Geometry: final body of the model. Coordinates: model frame, mm. A direction names the side the tool comes from. Coordinates: 2 decimals unless noted, no trailing zeros. Write each loop counter-clockwise with the first axis right and the second up, starting at its lowest first coordinate (ties: lowest second). Pieces come first, ordered by that corner, then holes. Notation, with made-up numbers: (-23.75, 77) - (12.25, 77) arc R27 ccw to (12.25, 113) - close; hole circle Ø10 at (51.25, 15). An arc over 180 degrees is marked (long way). Answer as a JSON object with one key per item and string values. Group by question number.
Item 1: Section B-B on y = -5. Return loops of the section in (x, z).
Item 2: Mould query, pull axis X, two halves, no side actions, for faces 1 (the flat face through (28, 0, -11)), 2 (the flat face through (-20, 0, -4)), 3 (the cylindrical face through (-22.7, -5.8, -10.6)). Classes: pulls with the +X half, pulls with the -X half, needs draft (parallel to the pull), parting line crosses it, or undercut.
Item 3: First-contact query: pin 1 Ø4 at (x, y) = (-25.5, 4) entering from -Z; pin 2 Ø10 at (y, z) = (4.5, -25.5) entering from +X; pin 3 Ø10 at (x, y) = (9, 1.5) entering from +Z. Flat tips, straight axial feed; report the tip coordinate or a pass-through.
Item 4: Set-up query: faces 4 (the cylindrical face through (0, 0, 3)), 5 (the flat face through (-20, 0, -26)), 6 (the flat face through (-18, -8, 0)). Return all of +Z, -Z, +X, -X, +Y, -Y with unobstructed straight access to the full face (end or side cutting, diameter ignored); none if empty.
Item 5: Line query: line 1 along Y through (x, z) = (-24.75, -11.4); line 2 along X through (y, z) = (-4.75, -30); line 3 along Z through (x, y) = (4, -2). Output: solid intervals per line, ascending. Write a range as from..to.
Item 6: Section D-D on x = 3. Return loops of the section in (y, z), and give its area (3 significant figures).
Item 7: Section C-C on z = -13. Return loops of the section in (x, y), and give its area (3 significant figures).
Item 8: Section A-A on x = -24.75. Return loops of the section in (y, z), and give its area (3 significant figures).
```python
from build123d import *

# Parameters (mm, degrees)
SKETCH1_W           = 40
SKETCH1_H           = 20
BOSS_EXTRUDE1_DEPTH = 40.5
SKETCH2_R           = 10
BOSS_EXTRUDE2_DEPTH = 7
SKETCH3_W           = 3.2
SKETCH3_H           = 20
BOSS_EXTRUDE3_DEPTH = 8
SKETCH4_W           = 3.2
SKETCH4_H           = 20
BOSS_EXTRUDE4_DEPTH = 8
SKETCH6_R           = 2.2
CUT_EXTRUDE1_DEPTH  = 8
SKETCH8_R           = 2.2
CUT_EXTRUDE3_DEPTH  = 8


with BuildPart() as part:
    # Sketch1 → Boss-Extrude1 (new body)
    with BuildSketch(Plane.XY):
        Rectangle(SKETCH1_W, SKETCH1_H)
    extrude(amount=-BOSS_EXTRUDE1_DEPTH)

    # Sketch2 → Boss-Extrude2 (add)
    with BuildSketch(Plane.XY):
        with Locations(Location((-10, 0, 0), (0, 0, 180))):
            Circle(SKETCH2_R)
    extrude(amount=BOSS_EXTRUDE2_DEPTH)

    # Sketch3 → Boss-Extrude3 (add)
    with BuildSketch(Plane.ZY.offset(20)):
        with Locations((-10.6, 0)):
            Rectangle(SKETCH3_W, SKETCH3_H)
    extrude(amount=BOSS_EXTRUDE3_DEPTH)

    # Sketch4 → Boss-Extrude4 (add)
    with BuildSketch(Plane(origin=(20, 0, 0), x_dir=(0, 0, -1), z_dir=(1, 0, 0))):
        with Locations((10.6, 0)):
            Rectangle(SKETCH4_W, SKETCH4_H)
    extrude(amount=BOSS_EXTRUDE4_DEPTH)

    # Sketch6 → Cut-Extrude1 (cut)
    with BuildSketch(Plane.XY.offset(-9)):
        with Locations((-24.75, 5)):
            Circle(SKETCH6_R)
        with Locations((-24.75, -5)):
            Circle(SKETCH6_R)
    extrude(amount=-CUT_EXTRUDE1_DEPTH, mode=Mode.SUBTRACT)

    # Sketch8 → Cut-Extrude3 (cut)
    with BuildSketch(Plane.XY.offset(-9)):
        with Locations((24.75, 5)):
            Circle(SKETCH8_R)
        with Locations((24.75, -5)):
            Circle(SKETCH8_R)
    extrude(amount=-CUT_EXTRUDE3_DEPTH, mode=Mode.SUBTRACT)


solid = part.part
```
Checks:
{
 "1": {"outline": "(-28, -12.2) - (-26.95, -12.2) - (-26.95, -9) - (-28, -9) - close; (-22.55, -12.2) - (-20, -12.2) - (-20, -40.5) - (20, -40.5) - (20, -12.2) - (22.55, -12.2) - (22.55, -9) - (20, -9) - (20, 0) - (-1.34, 0) - (-1.34, 7) - (-18.66, 7) - (-18.66, 0) - (-20, 0) - (-20, -9) - (-22.55, -9) - close; (26.95, -12.2) - (28, -12.2) - (28, -9) - (26.95, -9) - close"},
 "2": {"face 1": "pulls with the +X half", "face 2": "pulls with the -X half", "face 3": "undercut"},
 "3": {"pin 1": "z = -12.2", "pin 2": "x = 20", "pin 3": "z = 0"},
 "4": {"face 4": "+Z", "face 5": "-Z, -X, +Y, -Y", "face 6": "+Z, -X, -Y"},
 "5": {"line 1": "-10..-7.2, -2.8..2.8, 7.2..10", "line 2": "-20..20", "line 3": "-40.5..0"},
 "6": {"outline": "(-10, -40.5) - (10, -40.5) - (10, 0) - (-10, 0) - close", "area": "810 mm^2"},
 "7": {"outline": "(-20, -10) - (20, -10) - (20, 10) - (-20, 10) - close", "area": "800 mm^2"},
 "8": {"outline": "(-10, -12.2) - (-7.2, -12.2) - (-7.2, -9) - (-10, -9) - close; (-2.8, -12.2) - (2.8, -12.2) - (2.8, -9) - (-2.8, -9) - close; (7.2, -12.2) - (10, -12.2) - (10, -9) - (7.2, -9) - close", "area": "35.8 mm^2"}
}
